```python
from build123d import *

# Parameters (mm, degrees)
SKETCH1_R           = 5
BOSS_EXTRUDE1_DEPTH = 1
SKETCH2_R           = 4.4
BOSS_EXTRUDE2_DEPTH = 6
FILLET2_R           = 1
CHAMFER1_SIZE       = 0.75


with BuildPart() as part:
    # Sketch1 → Boss-Extrude1 (new body)
    with BuildSketch(Plane.XY):
        Circle(SKETCH1_R)
    extrude(amount=BOSS_EXTRUDE1_DEPTH)

    # Sketch2 → Boss-Extrude2 (add)
    with BuildSketch(Plane.XY.offset(1)):
        Circle(SKETCH2_R)
    extrude(amount=BOSS_EXTRUDE2_DEPTH)

    # Fillet2
    fillet2_edges = [part.edges().sort_by_distance(p)[0] for p in [
        (-4.4, 0, 7),
    ]]
    fillet(fillet2_edges, radius=FILLET2_R)

    # Chamfer1
    # the kernel refuses this chamfer: 0.75 mm, written as the material it takes off along each edge
    with BuildSketch(Plane(origin=(0, 0, 1), x_dir=(1, 0, 0), z_dir=(0, -1, 0))) as chamfer1_piece_1_section:
        Polygon((5 - CHAMFER1_SIZE, 0), (5, -CHAMFER1_SIZE), (5, 0), align=None)
    chamfer1_piece_1 = revolve(axis=Axis((0, 0, 1), (0, 0, 1)), mode=Mode.PRIVATE)
    chamfer1_piece_1 = chamfer1_piece_1 - Plane(origin=(0, 0, 0.553993393), x_dir=(1, 0, 0), z_dir=(0, 0, -1)) * Cylinder(4.4, 20, mode=Mode.PRIVATE)
    add(chamfer1_piece_1, mode=Mode.SUBTRACT)


solid = part.part
```
Build history of the part. All positions in model axes, mm. Round coordinates to 2 decimals unless told otherwise and drop trailing zeros. Loops run counter-clockwise (first coordinate to the right, second up) from the corner with the lowest first, then second, coordinate; pieces in that order, holes last.
Item 1: Pin check, flat tip, straight feed: P1, Ø3, axis at x = 2, z = 4.5, coming from the -Y side. Stop position of the tip, or through.
Item 2: Drill centre lines: line 1 along Z through (x, y) = (3.5, -1); line 2 along X through (y, z) = (2.25, 3.5); line 3 along Y through (x, z) = (-2, 3). Where is each one in solid material? Low to high.
Item 3: Saw through at A-A (x = 0). List the corners of the cut face in (y, z).
Item 4: Saw through at C-C (z = 1.5). List the corners of the cut face in (x, y), then the cut area to 3 significant figures.
Item 5: Two-plate mould, pull along Z, no slides. Class faces 1 (the face through (0, 0, 7)), 2 (the face through (0, 0, 0)): released by +Z, released by -Z, zero draft, split by the parting line, or undercut.
Worked answers:
1. P1: stops at y = -4.37
2. line 1: z = 0 to 6.97
2. line 2: x = -3.78 to 3.78
2. line 3: y = -3.92 to 3.92
3. outline: (-5, 0) - (5, 0) - (5, 0.25) - (4.4, 0.85) - (4.4, 6) arc R1 ccw to (3.4, 7) - (-3.4, 7) arc R1 ccw to (-4.4, 6) - (-4.4, 0.85) - (-5, 0.25) - close
4. outline: circle Ø8.8 at (0, 0)
4. area: 60.8 mm2
5. face 1: released by +Z
5. face 2: released by -Z
